Could you check a few things on this model? Use its own coordinates, in mm. A direction names the side the tool comes from. Round coordinates to 2 decimals unless told otherwise and drop trailing zeros. Loops run counter-clockwise (first coordinate to the right, second up) from the corner with the lowest first, then second, coordinate; pieces in that order, holes last. Notation, with made-up numbers: M 40,16.25 L 95,16.25 A30 ccw 95,50.25 Z; hole C 84,-11.75 d4. An arc over 180 degrees is marked long. One line per item, written item: value. Start each with the question number.
Q1. Please list where these lines run through material, in increasing order: line 1 along X through (y, z) = (24.5, -4.5); line 2 along Y through (x, z) = (6.5, -15.5); line 3 along X through (y, z) = (20, -14.25).
Q2. Thinking about a two-plate mould opening in Y: for faces 3 (the face through (-15.9, 9.3, 0)), 4 (the face through (-17.45, 24.8, -9.86)), 5 (the face through (-13.147, 5.964, -9.86)), 6 (the face through (-17.935, 24.986, -9.86)), which applies, released by +Y, released by -Y, zero draft, split by the parting line, or undercut?
Q3. I'm going to push flat-ended pins straight in: pin 1 Ø2 at (y, z) = (4, -15.5) entering from +X; pin 2 Ø4 at (y, z) = (9.5, -14.5) entering from -X; pin 3 Ø12 at (y, z) = (20.5, -5) entering from +X. Where does each tip first touch, or does it pass through?
Q4. Imagine slicing it at B-B (x = 0.75). Please give me the cut outline in (y, z), then the cut area to 3 significant figures.
Q5. Which directions (+Z, -Z, +X, -X, +Y, -Y) give clear straight access to the entire face, cutting with the end or side of a thin tool? Please do faces 1 (the face through (5, -0.25, -10)), 2 (the face through (5, 0.25, -10)).
Q6. Imagine slicing it at A-A (z = -6.75). Please give me the cut outline in (x, y).
from build123d import *

# Parameters (mm, degrees)
BOSS_EXTRUDE1_DEPTH = 20


with BuildPart() as part:
    # Sketch1 → Boss-Extrude1 (new body)
    with BuildSketch(Plane.XY):
        with BuildLine():
            Line((10, -0.25), (10, 0.25))
            Line((10, 0.25), (0, 0.25))
            ThreePointArc((0, 0.25), (-13.289004078, 6.117752441), (-17.905282596, 19.891572562))
            Line((-17.905282596, 19.891572562), (-16.982390424, 29.848894995))
            Line((-16.982390424, 29.848894995), (-17.480256546, 29.895039604))
            Line((-17.480256546, 29.895039604), (-18.403148718, 19.937717171))
            ThreePointArc((-18.403148718, 19.937717171), (-13.658512065, 5.780908489), (0, -0.25))
            Line((0, -0.25), (10, -0.25))
        make_face()
    extrude(amount=-BOSS_EXTRUDE1_DEPTH)


solid = part.part
Report:
1. line 1: x = -17.98 to -17.48
1. line 2: y = -0.25 to 0.25
1. line 3: x = -18.4 to -17.9
2. face 3: zero draft
2. face 4: undercut
2. face 5: undercut
2. face 6: released by +Y
3. pin 1: stops at x = -9.56
3. pin 2: stops at x = -17.21
3. pin 3: stops at x = -17.29
4. outline: M -0.25,-20 L 0.25,-20 L 0.25,0 L -0.25,0 Z
4. area: 10.0 mm²
5. face 1: +Z, -Z, +X, -X, -Y
5. face 2: +Z, -Z, +X, +Y
6. outline: M -18.4,19.94 A18.48 ccw 0,-0.25 L 10,-0.25 L 10,0.25 L 0,0.25 A17.98 cw -17.91,19.89 L -16.98,29.85 L -17.48,29.9 Z
